from build123d import *

# Parameters (mm, degrees)
F0_W      = 125
F0_H      = 100
F1_DEPTH  = 63.5
F3_D      = 3.7973
F3_DEPTH  = 10
F3_TIP    = 1.1408240143
F2_W      = 30.6147579104
F2_H      = 25.0281281769
F4_DEPTH  = 3
F5_R      = 2
F6_W      = 71.9727240503
F6_H      = 59.7681310028
F7_DEPTH  = 2
F9_DEPTH  = 5
F10_DEPTH = 5


with BuildPart() as f1:
    # F0 (on Top) → F1 (new body)
    with BuildSketch(Plane.XY):
        Rectangle(F0_W, F0_H)
    extrude(amount=F1_DEPTH)

    # F3
    with Locations(Plane(origin=(0, 50, 0), x_dir=(-1, 0, 0), z_dir=(0, 1, 0))):
        with Locations((-56.5, 32.5), (56.5, 57.5), (56.5, 6)):
            Hole(F3_D / 2, depth=F3_DEPTH)
            with Locations((0, 0, -(F3_DEPTH + F3_TIP / 2))):  # 118° drill point
                Cone(0, F3_D / 2, F3_TIP, mode=Mode.SUBTRACT)

    # F2 (on face) → F4 (join)
    with BuildSketch(Plane(origin=(0, 50, 0), x_dir=(-1, 0, 0), z_dir=(0, 1, 0))):
        with Locations((-36.4209739491, 27.976481244)):
            Rectangle(F2_W, F2_H)
    extrude(amount=F4_DEPTH)

    # F5
    f5_edges = [f1.edges().sort_by_distance(p)[0] for p in [
        (36.420974, 53, 40.490545),
        (51.728353, 53, 27.976481),
        (36.420974, 53, 15.462417),
        (21.113595, 53, 27.976481),
        (21.113595, 51.5, 40.490545),
        (21.113595, 51.5, 15.462417),
        (51.728353, 51.5, 40.490545),
        (51.728353, 51.5, 15.462417),
    ]]
    fillet(f5_edges, radius=F5_R)

    # F6 (on face) → F7 (cut)
    with BuildSketch(Plane.XY.offset(63.5)):
        with Locations((9.2756617814, -15.7460393384)):
            Rectangle(F6_W, F6_H)
    extrude(amount=-F7_DEPTH, mode=Mode.SUBTRACT)

    # F8 (on face) → F9 (cut)
    with BuildSketch(Plane(origin=(0, 50, 0), x_dir=(-1, 0, 0), z_dir=(0, 1, 0))):
        with BuildLine():
            Line((-7.6500625238, 55.638247937), (-9.9858876914, 55.638247937))
            ThreePointArc((-9.9858876914, 55.638247937), (-11.0465478632, 55.1989081087), (-11.4858876914, 54.138247937))
            Line((-11.4858876914, 54.138247937), (-11.4858876914, 7.0822326578))
            ThreePointArc((-11.4858876914, 7.0822326578), (-11.0465478632, 6.021572486), (-9.9858876914, 5.5822326578))
            Line((-9.9858876914, 5.5822326578), (-7.6500625238, 5.5822326578))
            ThreePointArc((-7.6500625238, 5.5822326578), (-6.589402352, 6.021572486), (-6.1500625238, 7.0822326578))
            Line((-6.1500625238, 7.0822326578), (-6.1500625238, 54.138247937))
            ThreePointArc((-6.1500625238, 54.138247937), (-6.589402352, 55.1989081087), (-7.6500625238, 55.638247937))
        make_face()
        with BuildLine():
            Line((2.3499374762, 55.638247937), (0.0141123086, 55.638247937))
            ThreePointArc((0.0141123086, 55.638247937), (-1.0465478632, 55.1989081087), (-1.4858876914, 54.138247937))
            Line((-1.4858876914, 54.138247937), (-1.4858876914, 7.0822326578))
            ThreePointArc((-1.4858876914, 7.0822326578), (-1.0465478632, 6.021572486), (0.0141123086, 5.5822326578))
            Line((0.0141123086, 5.5822326578), (2.3499374762, 5.5822326578))
            ThreePointArc((2.3499374762, 5.5822326578), (3.410597648, 6.021572486), (3.8499374762, 7.0822326578))
            Line((3.8499374762, 7.0822326578), (3.8499374762, 54.138247937))
            ThreePointArc((3.8499374762, 54.138247937), (3.410597648, 55.1989081087), (2.3499374762, 55.638247937))
        make_face()
        with BuildLine():
            Line((12.3499374762, 55.638247937), (10.0141123086, 55.638247937))
            ThreePointArc((10.0141123086, 55.638247937), (8.9534521368, 55.1989081087), (8.5141123086, 54.138247937))
            Line((8.5141123086, 54.138247937), (8.5141123086, 7.0822326578))
            ThreePointArc((8.5141123086, 7.0822326578), (8.9534521368, 6.021572486), (10.0141123086, 5.5822326578))
            Line((10.0141123086, 5.5822326578), (12.3499374762, 5.5822326578))
            ThreePointArc((12.3499374762, 5.5822326578), (13.410597648, 6.021572486), (13.8499374762, 7.0822326578))
            Line((13.8499374762, 7.0822326578), (13.8499374762, 54.138247937))
            ThreePointArc((13.8499374762, 54.138247937), (13.410597648, 55.1989081087), (12.3499374762, 55.638247937))
        make_face()
        with BuildLine():
            Line((22.3499374762, 55.638247937), (20.0141123086, 55.638247937))
            ThreePointArc((20.0141123086, 55.638247937), (18.9534521368, 55.1989081087), (18.5141123086, 54.138247937))
            Line((18.5141123086, 54.138247937), (18.5141123086, 7.0822326578))
            ThreePointArc((18.5141123086, 7.0822326578), (18.9534521368, 6.021572486), (20.0141123086, 5.5822326578))
            Line((20.0141123086, 5.5822326578), (22.3499374762, 5.5822326578))
            ThreePointArc((22.3499374762, 5.5822326578), (23.410597648, 6.021572486), (23.8499374762, 7.0822326578))
            Line((23.8499374762, 7.0822326578), (23.8499374762, 54.138247937))
            ThreePointArc((23.8499374762, 54.138247937), (23.410597648, 55.1989081087), (22.3499374762, 55.638247937))
        make_face()
        with BuildLine():
            Line((32.3499374762, 55.638247937), (30.0141123086, 55.638247937))
            ThreePointArc((30.0141123086, 55.638247937), (28.9534521368, 55.1989081087), (28.5141123086, 54.138247937))
            Line((28.5141123086, 54.138247937), (28.5141123086, 7.0822326578))
            ThreePointArc((28.5141123086, 7.0822326578), (28.9534521368, 6.021572486), (30.0141123086, 5.5822326578))
            Line((30.0141123086, 5.5822326578), (32.3499374762, 5.5822326578))
            ThreePointArc((32.3499374762, 5.5822326578), (33.410597648, 6.021572486), (33.8499374762, 7.0822326578))
            Line((33.8499374762, 7.0822326578), (33.8499374762, 54.138247937))
            ThreePointArc((33.8499374762, 54.138247937), (33.410597648, 55.1989081087), (32.3499374762, 55.638247937))
        make_face()
        with BuildLine():
            Line((42.3499374762, 55.638247937), (40.0141123086, 55.638247937))
            ThreePointArc((40.0141123086, 55.638247937), (38.9534521368, 55.1989081087), (38.5141123086, 54.138247937))
            Line((38.5141123086, 54.138247937), (38.5141123086, 7.0822326578))
            ThreePointArc((38.5141123086, 7.0822326578), (38.9534521368, 6.021572486), (40.0141123086, 5.5822326578))
            Line((40.0141123086, 5.5822326578), (42.3499374762, 5.5822326578))
            ThreePointArc((42.3499374762, 5.5822326578), (43.410597648, 6.021572486), (43.8499374762, 7.0822326578))
            Line((43.8499374762, 7.0822326578), (43.8499374762, 54.138247937))
            ThreePointArc((43.8499374762, 54.138247937), (43.410597648, 55.1989081087), (42.3499374762, 55.638247937))
        make_face()
    extrude(amount=-F9_DEPTH, mode=Mode.SUBTRACT)

    # F10 (cut): a face of the model
    f10_faces = [f1.faces().sort_by_distance(p)[0] for p in [
        (36.4209739491, 53, 27.976481244),
    ]]
    extrude(f10_faces, amount=-F10_DEPTH, mode=Mode.SUBTRACT)


solid = f1.part
Could you check a few things on this model? Use its own coordinates, in mm. A direction names the side the tool comes from. Coordinates: 2 decimals unless noted, no trailing zeros. Order: outer loops, then holes, each group sorted by start corner. A loop starts at its lowest first (then second) coordinate and runs counter-clockwise, first axis right, second up. Notation, with made-up numbers: (30.25, 15.5) -> (87.25, 15.5) arc R34 cw to (87.25, 48.5) -> close; hole circle Ø9 at (69, -36). An arc over 180 degrees is marked (long way). One line per item, written item: value. Start each with the question number.
1) We'd pull the mould along Z, two halves only. Please class faces 4 (the flat face through (-1, -50, 31)), 5 (the flat face through (-1, 1, 0)), 6 (the flat face through (-15, 23, 63.5)), 7 (the cylindrical face through (-58.007, 44.93, 56.345)): +Z half, -Z half, draft (parallel to the pull), parting line (faces both ways), or undercut.
2) Imagine slicing it at B-B on x = 40. List the corners of the cut face in (y, z) for me, plus the area to 3 significant figures.
3) Which directions (+Z, -Z, +X, -X, +Y, -Y) give clear straight access to the entire face, cutting with the end or side of a thin tool? Please do faces 1 (the flat face through (-18.514, 48, 31)), 2 (the flat face through (62.5, -1, 31)), 3 (the flat face through (9, -15, 61.5)).
4) If I drill on L1, parallel to Z at x = -56.5, y = 42.5; L2, parallel to X at y = 45, z = 57.5; L3, parallel to Y at x = -10.5, z = 43, over which ranges is the centre line in solid material (lowest first)? Write a range as [from, to].
5) Imagine slicing it at A-A on z = 46. List the corners of the cut face in (x, y) for me.
6) I'm going to push flat-ended pins straight in: pin 1 (12 mm diameter, centred on x = 13, z = 10.5, fed in from +Y); pin 2 (10.5 mm diameter, centred on x = 40.5, z = 28.5, fed in from +Y); pin 3 (0.8 mm diameter, centred on x = 40.5, y = 50.5, fed in from +Z). Where does each tip first touch, or does it pass through?
Answer list:
1. face 4: draft
1. face 5: -Z half
1. face 6: +Z half
1. face 7: undercut
2. outline: (-50, 0) -> (50, 0) -> (50, 15.46) -> (51, 15.46) arc R2 ccw to (53, 17.46) -> (48, 17.46) -> (48, 38.49) -> (53, 38.49) arc R2 ccw to (51, 40.49) -> (50, 40.49) -> (50, 63.5) -> (14.14, 63.5) -> (14.14, 61.5) -> (-45.63, 61.5) -> (-45.63, 63.5) -> (-50, 63.5) -> close
2. area: 6,200 mm2
3. face 1: +Y
3. face 2: +Z, -Z, +X, +Y, -Y
3. face 3: +Z
4. L1: z = [0, 4.1], [7.9, 55.6], [59.4, 63.5]
4. L2: x = [-62.5, -58.4], [-54.6, 62.5]
4. L3: y = [-50, 45]
5. outline: (-62.5, -50) -> (62.5, -50) -> (62.5, 50) -> (11.49, 50) -> (11.49, 45) -> (6.15, 45) -> (6.15, 50) -> (1.49, 50) -> (1.49, 45) -> (-3.85, 45) -> (-3.85, 50) -> (-8.51, 50) -> (-8.51, 45) -> (-13.85, 45) -> (-13.85, 50) -> (-18.51, 50) -> (-18.51, 45) -> (-23.85, 45) -> (-23.85, 50) -> (-28.51, 50) -> (-28.51, 45) -> (-33.85, 45) -> (-33.85, 50) -> (-38.51, 50) -> (-38.51, 45) -> (-43.85, 45) -> (-43.85, 50) -> (-62.5, 50) -> close
6. pin 1: stops at y = 50
6. pin 2: stops at y = 48
6. pin 3: stops at z = 40.49
